Geometry: see drawing. Coordinates: mm, zero at the bounding-box minimum. A direction names the side the tool comes from. Give positions to 0.01 mm unless a question says otherwise; leave off trailing zeros. Loops run counter-clockwise (first coordinate to the right, second up) from the corner with the lowest first, then second, coordinate; pieces in that order, holes last. Notation, with made-up numbers: (2.25, 71) -> (52.25, 71) arc R18 ccw to (52.25, 77) -> close; hole circle Ø6 at (2.25, 12). An arc over 180 degrees is marked (long way). One line per question, with ' | ' between items.
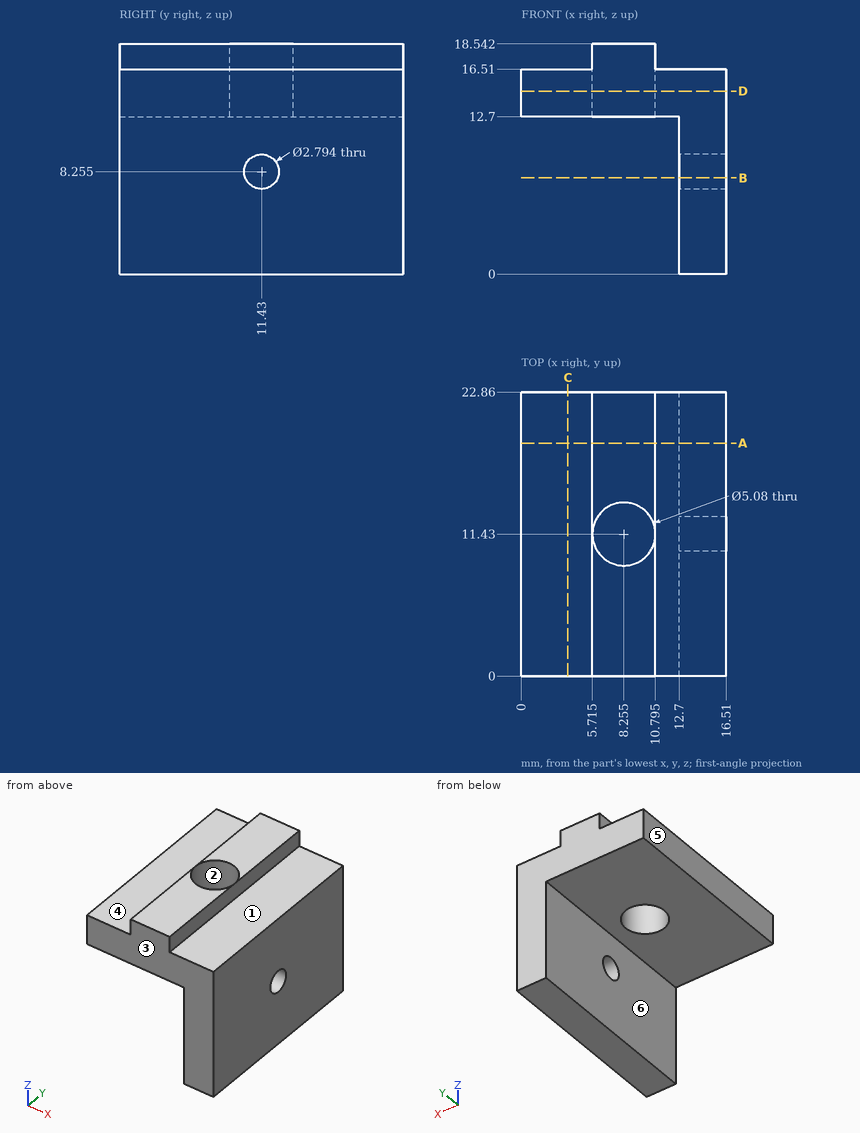
1. Pull-direction query (Y, two-part tool) for the marked faces 1, 2 and 3; classes: pulls with the +Y half, pulls with the -Y half, needs draft (parallel to the pull), parting line crosses it, or undercut.
Determined:
face 1: needs draft | face 2: undercut | face 3: pulls with the -Y half
2. Section query B-B (z = 7.75). Output: boundary loops of the cut face in (x, y), then the cut area to 3 significant figures.
Determined:
outline: (12.7, 0) -> (16.51, 0) -> (16.51, 10.13) -> (12.7, 10.13) -> close; (12.7, 12.73) -> (16.51, 12.73) -> (16.51, 22.86) -> (12.7, 22.86) -> close | area: 77.2 mm2
3. Section query A-A (y = 18.75). Output: boundary loops of the cut face in (x, z) (3 decimals).
Determined:
outline: (0, 12.7) -> (12.7, 12.7) -> (12.7, 0) -> (16.51, 0) -> (16.51, 16.51) -> (10.795, 16.51) -> (10.795, 18.542) -> (5.715, 18.542) -> (5.715, 16.51) -> (0, 16.51) -> close
4. Section query D-D (z = 14.75). Output: boundary loops of the cut face in (x, y) (3 decimals).
Determined:
outline: (0, 0) -> (16.51, 0) -> (16.51, 22.86) -> (0, 22.86) -> close; hole circle Ø5.08 at (8.255, 11.43)
5. Section query C-C (x = 3.75). Output: boundary loops of the cut face in (y, z), then the cut area to 3 significant figures.
Determined:
outline: (0, 12.7) -> (22.86, 12.7) -> (22.86, 16.51) -> (0, 16.51) -> close | area: 87.1 mm2
6. Reachability of the marked faces 4, 5 and 6 from +Z, -Z, +X, -X, +Y, -Y: full face, straight path, thin tool, end or side. Return the list, or none.
Determined:
face 4: +Z, -X, +Y, -Y | face 5: +Z, -Z, -X, +Y, -Y | face 6: -Z, -X, +Y, -Y
7. Pin query (flat end, axial travel): P1, Ø8, axis at y = 14.5, z = 5.5, coming from the -X side; P2, Ø1.6, axis at y = 8, z = 18, coming from the +X side (3 decimals); P3, Ø8, axis at x = 8.255, y = 11.43, coming from the -Z side; P4, Ø1, axis at x = 11.5, z = 12, coming from the -Y side. Return the tip coordinate at first contact, or that it passes through.
Determined:
P1: stops at x = 12.7 | P2: stops at x = 10.795 | P3: stops at z = 12.7 | P4: passes through
8. Ray query, line 1 along X through (y, z) = (11.43, 15.3) (3 decimals); line 2 along Z through (x, y) = (15.5, 4); line 3 along X through (y, z) = (3, 4.5). Return the intervals inside material, ascending. Write a range as from..to.
Determined:
line 1: x = 0..5.715, 10.795..16.51 | line 2: z = 0..16.51 | line 3: x = 12.7..16.51
